```python
from build123d import *

# Parameters (mm, degrees)
SKETCH1_W                = 20
SKETCH1_H                = 20
BOSS_EXTRUDE1_DEPTH      = 14.5
SKETCH2_R                = 7.5
BOSS_EXTRUDE2_DEPTH      = 3
F_8_0_8_DIAMETER_HOLE1_D = 8
CHAMFER1_SIZE            = 5
CHAMFER2_SIZE            = 2
CHAMFER3_SIZE            = 0.5


with BuildPart() as part:
    # Sketch1 → Boss-Extrude1 (new body)
    with BuildSketch(Plane(origin=(0, 0, 0), x_dir=(1, 0, 0), z_dir=(0, 1, 0))):
        Rectangle(SKETCH1_W, SKETCH1_H)
    extrude(amount=-BOSS_EXTRUDE1_DEPTH)

    # Sketch2 → Boss-Extrude2 (add)
    with BuildSketch(Plane(origin=(0, 0, 0), x_dir=(-1, 0, 0), z_dir=(0, 1, 0))):
        with Locations(Location((0, 0, 0), (0, 0, 90))):
            Circle(SKETCH2_R)
    extrude(amount=BOSS_EXTRUDE2_DEPTH)

    # Ø8.0 (8) Diameter Hole1 (through all)
    with Locations(Plane.XY.offset(10)):
        with Locations((0, -6)):
            Hole(F_8_0_8_DIAMETER_HOLE1_D / 2)

    # Chamfer1
    chamfer1_edges = [part.edges().sort_by_distance(p)[0] for p in [
        (-10, -14.5, 0),
        (10, -14.5, 0),
    ]]
    chamfer(chamfer1_edges, length=CHAMFER1_SIZE)

    # Chamfer2
    chamfer2_edges = [part.edges().sort_by_distance(p)[0] for p in [
        (-10, 0, 0),
        (10, 0, 0),
    ]]
    chamfer(chamfer2_edges, length=CHAMFER2_SIZE)

    # Chamfer3
    chamfer3_edges = [part.edges().sort_by_distance(p)[0] for p in [
        (4, -6, 10),
        (4, -6, -10),
    ]]
    chamfer(chamfer3_edges, length=CHAMFER3_SIZE)


solid = part.part
```
Design review of the part built by this model. Coordinates are the model's own, in mm. A direction names the side the tool comes from. Give positions to 0.01 mm unless a question says otherwise; leave off trailing zeros. Loops run counter-clockwise (first coordinate to the right, second up) from the corner with the lowest first, then second, coordinate; pieces in that order, holes last. Notation, with made-up numbers: M 71.25,14 L 122.25,14 A10 cw 122.25,20 Z; hole C 88.25,-2 d11. An arc over 180 degrees is marked long. Return JSON: item names as keys, results as strings. Group by question number.
Item 1: For probe 1 along Y at (x, z) = (0, 4); probe 2 along X at (y, z) = (-12, 0); probe 3 along Y at (x, z) = (-3.5, -7.5), list the stretches that pass through material, from the lowest coordinate up.
Item 2: We need section A-A (x = 0). Give the boundary of the cut face in (y, z).
Item 3: We need section D-D (z = 8.25). Give the boundary of the cut face in (x, y), and give its area (3 significant figures).
Item 4: Tool access review of faces 5 (the flat face through (-4, 0, -7)), 6 (the flat face through (-10, -6, 0)): name each direction out of +Z, -Z, +X, -X, +Y, -Y from which nothing blocks a thin tool from reaching the whole face with its end or side.
Item 5: We need section C-C (x = -6). Give the boundary of the cut face in (y, z).
Item 6: We need section B-B (z = 0). Give the boundary of the cut face in (x, y), and give its area (3 significant figures).
Item 7: Insertion check: pin 1 Ø4 at (y, z) = (-12.5, -2.5) entering from +X; pin 2 Ø1 at (x, y) = (6, 1) entering from -Z. Each pin has a flat end and moves straight along its axis. Give the tip position at first contact, or say it passes through.
Item 8: Mouldability with a two-part tool opening along X and no side actions: class faces 1 (the cylindrical face through (0.867, -9.905, -0.133)), 2 (the flat face through (0, -14.5, 0)), 3 (the flat face through (9, -1, 0)), 4 (the cylindrical face through (0.33, 1.479, -7.493)) as released by +X, released by -X, zero draft, split by the parting line, or undercut.
Output:
{
 "1": {"probe 1": "y = -14.5 to -10, -2 to 3", "probe 2": "x = -7.5 to 7.5", "probe 3": "y = -14.5 to -7.94, -4.06 to 0"},
 "2": {"outline": "M -14.5,-10 L -10.5,-10 L -10,-9.5 L -10,9.5 L -10.5,10 L -14.5,10 Z; M -2,-9.5 L -1.5,-10 L 0,-10 L 0,-7.5 L 3,-7.5 L 3,7.5 L 0,7.5 L 0,10 L -1.5,10 L -2,9.5 Z"},
 "3": {"outline": "M -10,-9.5 L -5,-14.5 L 5,-14.5 L 10,-9.5 L 10,-2 L 8,0 L -8,0 L -10,-2 Z; hole C 0,-6 d8", "area": "211 mm^2"},
 "4": {"face 5": "+Y", "face 6": "+Z, -Z, -X, +Y, -Y"},
 "5": {"outline": "M -13.5,-10 L 0,-10 L 0,-4.5 L 3,-4.5 L 3,4.5 L 0,4.5 L 0,10 L -13.5,10 Z"},
 "6": {"outline": "M -10,-9.5 L -5,-14.5 L 5,-14.5 L 10,-9.5 L 10,-2 L 8,0 L 7.5,0 L 7.5,3 L -7.5,3 L -7.5,0 L -8,0 L -10,-2 Z; hole C 0,-6 d8", "area": "256 mm^2"},
 "7": {"pin 1": "stops at x = 9", "pin 2": "stops at z = -5.1"},
 "8": {"face 1": "undercut", "face 2": "zero draft", "face 3": "released by +X", "face 4": "split by the parting line"}
}
